Can you work these out from the model? Positions are in its coordinate system, mm. A direction names the side the tool comes from. Coordinates: 2 decimals unless noted, no trailing zeros. Order: outer loops, then holes, each group sorted by start corner. A loop starts at its lowest first (then second) coordinate and runs counter-clockwise, first axis right, second up. Notation, with made-up numbers: (29.25, -14.5) -> (73.25, -14.5) arc R12 cw to (73.25, 4.5) -> close; hole circle Ø3 at (69, 29.25). An arc over 180 degrees is marked (long way). Write item = value, one per line.
```python
from build123d import *

# Parameters (mm, degrees)
F0_W     = 16.7
F0_H     = 16.7
F0_W_2   = 12.7
F0_H_2   = 12.7
F0_R     = 4.95
F1_DEPTH = 2
F2_DEPTH = 61.2
F3_R     = 0.5
F4_SIZE  = 3.8


with BuildPart() as f1:
    # F0 (on Front) → F1 (new body)
    with BuildSketch(Plane.XZ):
        with Locations((-2.257177, -4.186354)):
            Rectangle(F0_W, F0_H)
        with Locations((-2.257177, -4.186354)):
            Rectangle(F0_W_2, F0_H_2, mode=Mode.SUBTRACT)
        with Locations((-2.257177, -4.186354)):
            Rectangle(F0_W_2, F0_H_2)
        with Locations((-2.257177, -4.186354)):
            Circle(F0_R, mode=Mode.SUBTRACT)
    extrude(amount=F1_DEPTH)

    # F0 (on Front) → F2 (join)
    with BuildSketch(Plane.XZ):
        with Locations((-2.257177, -4.186354)):
            Rectangle(F0_W_2, F0_H_2)
        with Locations((-2.257177, -4.186354)):
            Circle(F0_R, mode=Mode.SUBTRACT)
    extrude(amount=-F2_DEPTH)

    # F3
    f3_edges = [f1.edges().sort_by_distance(p)[0] for p in [
        (-10.607177, -1, 4.163646),
        (6.092823, -1, 4.163646),
        (6.092823, -1, -12.536354),
        (-10.607177, -1, -12.536354),
    ]]
    fillet(f3_edges, radius=F3_R)

    # F4
    f4_edges = [f1.edges().sort_by_distance(p)[0] for p in [
        (-8.607177, 30.6, -10.536354),
        (-8.607177, 30.6, 2.163646),
        (4.092823, 30.6, -10.536354),
        (4.092823, 30.6, 2.163646),
    ]]
    chamfer(f4_edges, length=F4_SIZE)


solid = f1.part
```
Item 1: If we mould it in two halves opening along X, with no side actions, what happens to faces 1 (the cylindrical face through (2.315, 30.042, -6.082)), 2 (the flat face through (-2, 30, -10.536)), 3 (the flat face through (-6.681, 30.172, -8.663))? For each: pulls with the +X half, pulls with the -X half, needs draft (parallel to the pull), parting line crosses it, or undercut.
A:
face_1 = undercut
face_2 = needs draft
face_3 = pulls with the -X half
Item 2: If I drill on probe 1 along X at (y, z) = (43.5, -4); probe 2 along X at (y, z) = (56.5, -8); probe 3 along Y at (x, z) = (4.5, -11.25), over which ranges is the centre line in solid material (lowest first)?
A:
probe_1 = -8.61 to -7.2, 2.69 to 4.09
probe_2 = -7.34 to -5.41, 0.9 to 2.83
probe_3 = -2 to 0
Item 3: I want a section at B-B, the plane z = -8. Please give me the cut outline in (x, y).
A:
outline = (-10.61, -2) -> (-5.41, -2) -> (-5.41, 61.2) -> (-7.34, 61.2) -> (-7.34, 0) -> (-10.61, 0) -> close; (0.9, -2) -> (6.09, -2) -> (6.09, 0) -> (2.83, 0) -> (2.83, 61.2) -> (0.9, 61.2) -> close
Item 4: I want a section at D-D, the plane x = 3.5. Please give me the cut outline in (y, z).
A:
outline = (-2, -12.54) -> (0, -12.54) -> (0, -7.33) -> (61.2, -7.33) -> (61.2, -1.04) -> (0, -1.04) -> (0, 4.16) -> (-2, 4.16) -> close
Item 5: I want a section at A-A, the plane x = -2.25. Please give me the cut outline in (y, z).
A:
outline = (-2, -12.54) -> (0, -12.54) -> (0, -10.54) -> (61.2, -10.54) -> (61.2, -9.14) -> (-2, -9.14) -> close; (-2, 0.76) -> (61.2, 0.76) -> (61.2, 2.16) -> (0, 2.16) -> (0, 4.16) -> (-2, 4.16) -> close
Item 6: I want a section at C-C, the plane y = 11.5. Please give me the cut outline in (x, z), plus the area to 3 significant figures.
A:
outline = (-8.61, -6.74) -> (-4.81, -10.54) -> (0.29, -10.54) -> (4.09, -6.74) -> (4.09, -1.64) -> (0.29, 2.16) -> (-4.81, 2.16) -> (-8.61, -1.64) -> close; hole circle Ø9.9 at (-2.26, -4.19)
area = 55.4 mm2
Item 7: I'm going to push flat-ended pins straight in: P1, Ø4, axis at x = -5, y = 42.5, coming from the -Z side; P2, Ø5.5, axis at y = 35.5, z = -3, coming from the +X side; P3, Ø3, axis at y = 18.5, z = 2.5, coming from the -X side; P4, Ø8, axis at x = -2.26, z = -4.19, coming from the -Y side (3 decimals). Where does each tip first touch, or does it pass through?
A:
P1 = -10.54
P2 = 4.09
P3 = -5.97
P4 = through
Item 8: For faces 4 (the flat face through (4.093, 30, -4)), 5 (the flat face through (-8.607, 30, -4)), 6 (the flat face through (2.219, 30.172, 0.237)), 7 (the flat face through (-6, 0, -10)), 8 (the flat face through (-2, 30, 2.164)), which set-ups out of +Z, -Z, +X, -X, +Y, -Y let a thin tool reach every point of the face, with its end or its side?
A:
face_4 = +Z, -Z, +X, +Y
face_5 = +Z, -Z, -X, +Y
face_6 = +Z, +X, +Y
face_7 = +Y
face_8 = +Z, +X, -X, +Y
